For this review, take the finished solid that the model builds, in its own axes (mm). A direction names the side the tool comes from. Give positions to 0.01 mm unless a question says otherwise; leave off trailing zeros. Loops run counter-clockwise (first coordinate to the right, second up) from the corner with the lowest first, then second, coordinate; pieces in that order, holes last.
```python
from build123d import *

# Parameters (mm, degrees)
PAD_DEPTH       = 11
POCKET_DEPTH    = 5
SKETCH003_R     = 1.05
POCKET001_DEPTH = 5
FILLET_R        = 1
FILLET001_R     = 1
FILLET002_R     = 1
SKETCH004_R     = 1
POCKET002_DEPTH = 5


with BuildPart() as part:
    # Sketch → Pad (new body)
    with BuildSketch(Plane.XY):
        Polygon((0, 0), (-5, 0), (-5, -3), (3, -3), (3, 24), (0, 24), align=None)
    extrude(amount=PAD_DEPTH)

    # Sketch002 (on Face6 of Pad) → Pocket (cut)
    with BuildSketch(Plane(origin=(0, 0, 0), x_dir=(0, -1, 0), z_dir=(-1, 0, 0))):
        Polygon((-24, 10.051275), (-24, 5.051275), (-14, 5.051275), (-14, 13.051275), (-24, 13.051275), align=None)
    extrude(amount=-POCKET_DEPTH, mode=Mode.SUBTRACT)

    # Sketch003 (on Face2 of Pocket) → Pocket001 (cut)
    with BuildSketch(Plane(origin=(0, 0, 0), x_dir=(0, -1, 0), z_dir=(-1, 0, 0))):
        with Locations((-22.2, 2.1)):
            Circle(SKETCH003_R)
    extrude(amount=-POCKET001_DEPTH, mode=Mode.SUBTRACT)

    # Fillet
    fillet_edges = [part.edges().sort_by_distance(p)[0] for p in [
        (0, 0, 5.5),
    ]]
    fillet(fillet_edges, radius=FILLET_R)

    # Fillet001
    fillet001_edges = [part.edges().sort_by_distance(p)[0] for p in [
        (-5, -1.5, 0),
    ]]
    fillet(fillet001_edges, radius=FILLET001_R)

    # Fillet002
    fillet002_edges = [part.edges().sort_by_distance(p)[0] for p in [
        (-5, -1.5, 11),
    ]]
    fillet(fillet002_edges, radius=FILLET002_R)

    # Sketch004 (on Face1 of Fillet002) → Pocket002 (cut)
    with BuildSketch(Plane(origin=(0, 0, 0), x_dir=(-1, 0, 0), z_dir=(0, 1, 0))):
        with Locations((3, 9)):
            Circle(SKETCH004_R)
        with Locations((3, 2)):
            Circle(SKETCH004_R)
    extrude(amount=-POCKET002_DEPTH, mode=Mode.SUBTRACT)


solid = part.part
```
Q1. Consider section D-D on x = 0.5. Give the boundary of the cut face in (y, z).
Answers:
outline: (-3, 0) - (24, 0) - (24, 5.05) - (14, 5.05) - (14, 11) - (-3, 11) - close; hole circle Ø2.1 at (22.2, 2.1)
Q2. For pin 1 Ø4 at (x, z) = (-3, 2) entering from +Y; pin 2 Ø2.5 at (x, y) = (2, 21) entering from +Z; pin 3 Ø1.5 at (x, z) = (1, 8.5) entering from +Y; pin 4 Ø2.5 at (y, z) = (22.2, 2.1) entering from +X, all flat-tipped, find the tip position at first contact; note any pin that passes through.
Answers:
pin 1: stops at y = 0
pin 2: stops at z = 5.05
pin 3: stops at y = 14
pin 4: stops at x = 3
Q3. Consider section B-B on z = 9. Give the boundary of the cut face in (x, y).
Answers:
outline: (-5, -3) - (-4, -3) - (-4, 0) - (-5, 0) - close; (-2, -3) - (3, -3) - (3, 14) - (0, 14) - (0, 1) arc R1 cw to (-1, 0) - (-2, 0) - close
Q4. For probe 1 along Z at (x, y) = (-3, -1.5); probe 2 along Z at (x, y) = (2.1, 22.2); probe 3 along Y at (x, z) = (-2, 2.75), list the stretches that pass through material, from the lowest coordinate up.
Answers:
probe 1: z = 0 to 1, 3 to 8, 10 to 11
probe 2: z = 0 to 1.05, 3.15 to 5.05
probe 3: y = -3 to 0
Q5. Mouldability with a two-part tool opening along Y and no side actions: class faces 1 (the cylindrical face through (-3, -1, 10)), 2 (the cylindrical face through (1.48, 23.25, 2.15)), 3 (the flat face through (-3, 0, 5)) as +Y half, -Y half, draft (parallel to the pull), parting line (faces both ways), or undercut.
Answers:
face 1: draft
face 2: undercut
face 3: +Y half
Q6. Machinability: for faces 4 (the flat face through (2, 24, 2)), 5 (the flat face through (0, 10, 4)), 6 (the flat face through (1, 14, 8)), which of the approach directions +Z, -Z, +X, -X, +Y, -Y give a long, thin tool a straight path to every point of the face, cutting with its end or side? Answer none if there is none.
Answers:
face 4: +Z, -Z, +X, -X, +Y
face 5: +Z, -Z, -X, +Y
face 6: +Z, +X, -X, +Y
Q7. Consider section C-C on y = 22.2. Give the boundary of the cut face in (x, z).
Answers:
outline: (0, 0) - (3, 0) - (3, 1.05) - (0, 1.05) - close; (0, 3.15) - (3, 3.15) - (3, 5.05) - (0, 5.05) - close
Q8. Consider section A-A on x = -3. Give the boundary of the cut face in (y, z).
Answers:
outline: (-3, 0) - (0, 0) - (0, 1) - (-3, 1) - close; (-3, 3) - (0, 3) - (0, 8) - (-3, 8) - close; (-3, 10) - (0, 10) - (0, 11) - (-3, 11) - close
